Model file for the job. Use its own axes, mm. A direction names the side the tool comes from. Round coordinates to 2 decimals unless told otherwise and drop trailing zeros. Order: outer loops, then holes, each group sorted by start corner. A loop starts at its lowest first (then second) coordinate and runs counter-clockwise, first axis right, second up. Notation, with made-up numbers: (-4, 34.25) - (52, 34.25) arc R22 cw to (52, 68.25) - close; hole circle Ø10 at (31.5, 51). An arc over 180 degrees is marked (long way). Put each result on its own line as item: value. Start each with the question number.
Item 1: Pin check, flat tip, straight feed: pin 1 Ø6.5 at (x, z) = (28.01, 18.6) entering from +Y. Stop position of the tip, or through.
Item 2: Which spindle directions (+Z, -Z, +X, -X, +Y, -Y) get a long thin tool onto all of the face, cutting with end or side? Do faces 1 (the face through (-1, 0, 189)), 2 (the face through (-14, -12, 261)). Say none if no direction does.
Item 3: Saw through at A-A on z = 362. List the corners of the cut face in (x, y).
Item 4: Probe probe 1 along X at (y, z) = (-4.75, 252); probe 2 along X at (y, z) = (-3, 26); probe 3 along Z at (x, y) = (33, -3.25). List the from-to ranges inside material, lowest first.
Item 5: Mould opens along X. For faces 3 (the face through (-1, -12, 411.096)), 4 (the face through (-36, -12, 372)), 5 (the face through (-55, -12, 183)) say: pulls with the +X half, pulls with the -X half, needs draft (parallel to the pull), parting line crosses it, or undercut.
```python
from build123d import *

# Parameters (mm, degrees)
F0_W     = 110
F0_H     = 450
F0_R     = 2.5
F0_R_2   = 2.6
F0_R_3   = 3.25
F0_W_2   = 72
F0_H_2   = 52
F1_DEPTH = 25


with BuildPart() as f1:
    # F0 (on Front) → F1 (new body)
    with BuildSketch(Plane.XZ):
        with Locations((0, 186.095581)):
            Rectangle(F0_W, F0_H)
        with Locations((-28.011849, 3.589829)):
            Circle(F0_R, mode=Mode.SUBTRACT)
        with Locations((-29, 11.095581)):
            Circle(F0_R, mode=Mode.SUBTRACT)
        with Locations((-28.011849, 18.601333)):
            Circle(F0_R, mode=Mode.SUBTRACT)
        with Locations((-14.5, -14.019156)):
            Circle(F0_R, mode=Mode.SUBTRACT)
        with Locations((-25.114737, -3.404419)):
            Circle(F0_R, mode=Mode.SUBTRACT)
        with Locations((-20.506097, -9.410516)):
            Circle(F0_R, mode=Mode.SUBTRACT)
        with Locations((-7.505752, -16.916268)):
            Circle(F0_R, mode=Mode.SUBTRACT)
        with Locations((-25.114737, 25.595581)):
            Circle(F0_R, mode=Mode.SUBTRACT)
        with Locations((-20.506097, 31.601678)):
            Circle(F0_R, mode=Mode.SUBTRACT)
        with Locations((-14.5, 36.210318)):
            Circle(F0_R, mode=Mode.SUBTRACT)
        with Locations((-7.505752, 39.10743)):
            Circle(F0_R, mode=Mode.SUBTRACT)
        with Locations((-10, 67.095581)):
            Circle(F0_R_2, mode=Mode.SUBTRACT)
        with Locations((-30, 111.095581)):
            Circle(F0_R_3, mode=Mode.SUBTRACT)
        with Locations((0, -17.904419)):
            Circle(F0_R, mode=Mode.SUBTRACT)
        with Locations((7.505752, -16.916268)):
            Circle(F0_R, mode=Mode.SUBTRACT)
        with Locations((14.5, -14.019156)):
            Circle(F0_R, mode=Mode.SUBTRACT)
        with Locations((20.506097, -9.410516)):
            Circle(F0_R, mode=Mode.SUBTRACT)
        with Locations((25.114737, -3.404419)):
            Circle(F0_R, mode=Mode.SUBTRACT)
        with Locations((0, 40.095581)):
            Circle(F0_R, mode=Mode.SUBTRACT)
        with Locations((7.505752, 39.10743)):
            Circle(F0_R, mode=Mode.SUBTRACT)
        with Locations((10, 67.095581)):
            Circle(F0_R_2, mode=Mode.SUBTRACT)
        with Locations((14.5, 36.210318)):
            Circle(F0_R, mode=Mode.SUBTRACT)
        with Locations((20.506097, 31.601678)):
            Circle(F0_R, mode=Mode.SUBTRACT)
        with Locations((25.114737, 25.595581)):
            Circle(F0_R, mode=Mode.SUBTRACT)
        with Locations((28.011849, 3.589829)):
            Circle(F0_R, mode=Mode.SUBTRACT)
        with Locations((29, 11.095581)):
            Circle(F0_R, mode=Mode.SUBTRACT)
        with Locations((28.011849, 18.601333)):
            Circle(F0_R, mode=Mode.SUBTRACT)
        with Locations((30, 111.095581)):
            Circle(F0_R_3, mode=Mode.SUBTRACT)
        with BuildLine():
            Line((-26, 231.095581), (-26, 289.095581))
            ThreePointArc((-26, 289.095581), (-24.242641, 293.338222), (-20, 295.095581))
            ThreePointArc((-20, 295.095581), (-15.757359, 293.338222), (-14, 289.095581))
            Line((-14, 289.095581), (-14, 231.095581))
            ThreePointArc((-14, 231.095581), (-15.757359, 226.85294), (-20, 225.095581))
            ThreePointArc((-20, 225.095581), (-24.242641, 226.85294), (-26, 231.095581))
        make_face(mode=Mode.SUBTRACT)
        with Locations((-10, 329.095581)):
            Circle(F0_R_2, mode=Mode.SUBTRACT)
        with BuildLine():
            Line((14, 231.095581), (14, 289.095581))
            ThreePointArc((14, 289.095581), (15.757359, 293.338222), (20, 295.095581))
            ThreePointArc((20, 295.095581), (24.242641, 293.338222), (26, 289.095581))
            Line((26, 289.095581), (26, 231.095581))
            ThreePointArc((26, 231.095581), (24.242641, 226.85294), (20, 225.095581))
            ThreePointArc((20, 225.095581), (15.757359, 226.85294), (14, 231.095581))
        make_face(mode=Mode.SUBTRACT)
        with Locations((10, 329.095581)):
            Circle(F0_R_2, mode=Mode.SUBTRACT)
        with Locations((0, 372.095581)):
            Rectangle(F0_W_2, F0_H_2, mode=Mode.SUBTRACT)
    extrude(amount=F1_DEPTH)


solid = f1.part
```
Results found:
1. pin 1: stops at y = 0
2. face 1: +Z, -Z, +X, -X, +Y
2. face 2: +Y, -Y
3. outline: (-55, -25) - (-36, -25) - (-36, 0) - (-55, 0) - close; (36, -25) - (55, -25) - (55, 0) - (36, 0) - close
4. probe 1: x = -55 to -26, -14 to 14, 26 to 55
4. probe 2: x = -55 to -27.58, -22.65 to 22.65, 27.58 to 55
4. probe 3: z = -38.9 to 109.85, 112.35 to 346.1, 398.1 to 411.1
5. face 3: needs draft
5. face 4: undercut
5. face 5: pulls with the -X half
